```python
from build123d import *

# Parameters (mm, degrees)
F0_R     = 5
F0_R_2   = 1.5
F1_DEPTH = 2
F2_R     = 4
F2_R_2   = 2.5
F3_DEPTH = 0.25
F4_R     = 4
F4_R_2   = 2.5
F5_DEPTH = 0.25


with BuildPart() as f1:
    # F0 (on Front) → F1 (new body, symmetric)
    with BuildSketch(Plane.XZ):
        Circle(F0_R)
        Circle(F0_R_2, mode=Mode.SUBTRACT)
    extrude(amount=F1_DEPTH, both=True)

    # F2 (on face) → F3 (cut)
    with BuildSketch(Plane.XZ.offset(2)):
        Circle(F2_R)
        Circle(F2_R_2, mode=Mode.SUBTRACT)
    extrude(amount=-F3_DEPTH, mode=Mode.SUBTRACT)

    # F4 (on face) → F5 (cut)
    with BuildSketch(Plane(origin=(0, 2, 0), x_dir=(-1, 0, 0), z_dir=(0, 1, 0))):
        Circle(F4_R)
        Circle(F4_R_2, mode=Mode.SUBTRACT)
    extrude(amount=-F5_DEPTH, mode=Mode.SUBTRACT)


solid = f1.part
```
Could you check a few things on this model? Use its own coordinates, in mm. A direction names the side the tool comes from. Round coordinates to 2 decimals unless told otherwise and drop trailing zeros. Loops run counter-clockwise (first coordinate to the right, second up) from the corner with the lowest first, then second, coordinate; pieces in that order, holes last. Notation, with made-up numbers: M -37.5,63.25 L 8.5,63.25 A6 cw 8.5,74.25 Z; hole C 76.5,70 d7. An arc over 180 degrees is marked long. Put each result on its own line as item: value.
Q1. Imagine slicing it at B-B (x = 0). Write out the boundary of the cut face in (y, z), then the cut area to 3 significant figures.
Check result:
outline: M -2,-5 L 2,-5 L 2,-4 L 1.75,-4 L 1.75,-2.5 L 2,-2.5 L 2,-1.5 L -2,-1.5 L -2,-2.5 L -1.75,-2.5 L -1.75,-4 L -2,-4 Z; M -2,1.5 L 2,1.5 L 2,2.5 L 1.75,2.5 L 1.75,4 L 2,4 L 2,5 L -2,5 L -2,4 L -1.75,4 L -1.75,2.5 L -2,2.5 Z
area: 26.5 mm2
Q2. Imagine slicing it at A-A (z = 0). Write out the boundary of the cut face in (x, y), then the cut area to 3 significant figures.
Check result:
outline: M -5,-2 L -4,-2 L -4,-1.75 L -2.5,-1.75 L -2.5,-2 L -1.5,-2 L -1.5,2 L -2.5,2 L -2.5,1.75 L -4,1.75 L -4,2 L -5,2 Z; M 1.5,-2 L 2.5,-2 L 2.5,-1.75 L 4,-1.75 L 4,-2 L 5,-2 L 5,2 L 4,2 L 4,1.75 L 2.5,1.75 L 2.5,2 L 1.5,2 Z
area: 26.5 mm2
Q3. Thinking about a two-plate mould opening in Z: for faces 3 (the face through (2, -1.75, 2)), 4 (the face through (-1.08, -0.03, -4.88)), 5 (the face through (2, 2, 0)), 6 (the face through (-1.5, 0.03, 0.07)), which applies, released by +Z, released by -Z, zero draft, split by the parting line, or undercut?
Check result:
face 3: undercut
face 4: split by the parting line
face 5: zero draft
face 6: undercut
Q4. I need wall thicknesses on probe 1 along Z at (x, y) = (0, 1.95); probe 2 along Z at (x, y) = (0, 1); probe 3 along Y at (x, z) = (3, -1.25). Which ranges of each line are inside material? Lowest first, please.
Check result:
probe 1: -5 to -4, -2.5 to -1.5, 1.5 to 2.5, 4 to 5
probe 2: -5 to -1.5, 1.5 to 5
probe 3: -1.75 to 1.75
Q5. Imagine slicing it at C-C (y = -0.75). Write out the boundary of the cut face in (x, z), then the cut area to 3 significant figures.
Check result:
outline: C 0,0 d10; hole C 0,0 d3
area: 71.5 mm2
Q6. Imagine slicing it at D-D (x = 2.25). Write out the boundary of the cut face in (y, z), then the cut area to 3 significant figures.
Check result:
outline: M -2,-4.47 L 2,-4.47 L 2,-3.31 L 1.75,-3.31 L 1.75,-1.09 L 2,-1.09 L 2,1.09 L 1.75,1.09 L 1.75,3.31 L 2,3.31 L 2,4.47 L -2,4.47 L -2,3.31 L -1.75,3.31 L -1.75,1.09 L -2,1.09 L -2,-1.09 L -1.75,-1.09 L -1.75,-3.31 L -2,-3.31 Z
area: 33.5 mm2
Q7. For pin 1 (1 mm diameter, centred on y = -0.5, z = 2.5, fed in from +X), with a flat end and sliding along its axis, tell me the tip position at first contact or that it passes through.
Check result:
pin 1: x = 4.58
Q8. On a 3-axis mill with a long thin cutter (end or side, diameter ignored), from which of +Z, -Z, +X, -X, +Y, -Y can I reach the whole of each face in a straight line? I mean faces 1 (the face through (-2, 1.75, 2)), 2 (the face through (2, -2, 0)). Say none if no direction works.
Check result:
face 1: +Y
face 2: +Z, -Z, +X, -X, -Y
